CAD build for the part. Positions are in the model's coordinates, mm. A direction names the side the tool comes from. Coordinates: 2 decimals unless noted, no trailing zeros. Order: outer loops, then holes, each group sorted by start corner. A loop starts at its lowest first (then second) coordinate and runs counter-clockwise, first axis right, second up.
from build123d import *

# Parameters (mm, degrees)
SKETCH1_R           = 2.5
BOSS_EXTRUDE1_DEPTH = 3.18
CUT_EXTRUDE1_DEPTH  = 147.499595989
FILLET1_R           = 10


with BuildPart() as part:
    # Sketch1 → Boss-Extrude1 (new body)
    with BuildSketch(Plane(origin=(0, 0, 0), x_dir=(1, 0, 0), z_dir=(0, 1, 0))):
        Polygon((0, 0), (40, 0), (90, 0), (90, 40), (90, 75.550937794), (90, 115.550937794), (-50, 115.550937794), (-50, 0), align=None)
        with Locations(Location((-35, 105.550937794, 0), (0, 0, 90))):
            Circle(SKETCH1_R, mode=Mode.SUBTRACT)
        with Locations(Location((75, 105.550937794, 0), (0, 0, 90))):
            Circle(SKETCH1_R, mode=Mode.SUBTRACT)
        with Locations(Location((20, 85.550937794, 0), (0, 0, 90))):
            Circle(SKETCH1_R, mode=Mode.SUBTRACT)
        with Locations(Location((10, 7.5, 0), (0, 0, 90))):
            Circle(SKETCH1_R, mode=Mode.SUBTRACT)
        with Locations(Location((30, 7.5, 0), (0, 0, 90))):
            Circle(SKETCH1_R, mode=Mode.SUBTRACT)
        with Locations(Location((10, 32, 0), (0, 0, 90))):
            Circle(SKETCH1_R, mode=Mode.SUBTRACT)
        with Locations(Location((30, 32, 0), (0, 0, 90))):
            Circle(SKETCH1_R, mode=Mode.SUBTRACT)
    extrude(amount=BOSS_EXTRUDE1_DEPTH)

    # Sketch3 → Cut-Extrude1 (cut, through all)
    with BuildSketch(Plane.XZ):
        Polygon((90, -75.550937794), (50, -37.231146138), (50, 0), (90, 0), (90, -37.231146138), align=None)
        Polygon((-10, -37.231146138), (-50, -75.550937794), (-50, -37.231146138), (-50, 0), (-10, 0), align=None)
    extrude(amount=-CUT_EXTRUDE1_DEPTH, mode=Mode.SUBTRACT)

    # Fillet1
    fillet1_edges = [part.edges().sort_by_distance(p)[0] for p in [
        (-50, 1.59, -115.550937794),
        (90, 1.59, -115.550937794),
        (90, 1.59, -75.550937794),
        (50, 1.59, -37.231146138),
        (50, 1.59, 0),
        (-10, 1.59, 0),
        (-10, 1.59, -37.231146138),
        (-50, 1.59, -75.550937794),
    ]]
    fillet(fillet1_edges, radius=FILLET1_R)


solid = part.part
1) Two-plate mould, pull along Z, no slides. Class faces 1 (the cylindrical face through (27.52, 1.57, -31.67)), 2 (the flat face through (20, 2, 0)), 3 (the flat face through (-10, 2, -21)): released by +Z, released by -Z, zero draft, split by the parting line, or undercut.
2) Slice it at A-A (x = 30). List the corners of the cut face in (y, z).
3) Which spindle directions (+Z, -Z, +X, -X, +Y, -Y) get a long thin tool onto all of the face, cutting with end or side? Do faces 4 (the flat face through (50, 2, -22)), 5 (the flat face through (-50, 2, -93)). Say none if no direction does.
4) Slice it at C-C (z = -7.5). List the corners of the cut face in (x, y), plus the area to 3 significant figures.
5) Drill centre lines: probe 1 along Z at (x, y) = (30, 2.25); probe 2 along X at (y, z) = (1.7, -32); probe 3 along X at (y, z) = (2.55, -7). Where is each one in solid material? Low to high.
6) Slice it at B-B (y = 2.35). List the corners of the cut face in (x, z).
7) Slice it at D-D (x = -35). List the corners of the cut face in (y, z).
Worked out:
1. face 1: undercut
1. face 2: released by +Z
1. face 3: zero draft
2. outline: (0, -115.55) - (3.18, -115.55) - (3.18, -34.5) - (0, -34.5) - close; (0, -29.5) - (3.18, -29.5) - (3.18, -10) - (0, -10) - close; (0, -5) - (3.18, -5) - (3.18, 0) - (0, 0) - close
3. face 4: +Z, +X, +Y, -Y
3. face 5: +Z, -Z, -X, +Y, -Y
4. outline: (-9.68, 0) - (7.5, 0) - (7.5, 3.18) - (-9.68, 3.18) - close; (12.5, 0) - (27.5, 0) - (27.5, 3.18) - (12.5, 3.18) - close; (32.5, 0) - (49.68, 0) - (49.68, 3.18) - (32.5, 3.18) - close
4. area: 157 mm2
5. probe 1: z = -115.55 to -34.5, -29.5 to -10, -5 to 0
5. probe 2: x = -10 to 7.5, 12.5 to 27.5, 32.5 to 50
5. probe 3: x = -9.54 to 7.55, 12.45 to 27.55, 32.45 to 49.54
6. outline: (-50, -105.55) arc R10 ccw to (-40, -115.55) - (80, -115.55) arc R10 ccw to (90, -105.55) - (90, -79.82) arc R10 ccw to (86.92, -72.6) - (53.08, -40.18) arc R10 cw to (50, -32.96) - (50, -10) arc R10 ccw to (40, 0) - (0, 0) arc R10 ccw to (-10, -10) - (-10, -32.96) arc R10 cw to (-13.08, -40.18) - (-46.92, -72.6) arc R10 ccw to (-50, -79.82) - close; hole circle Ø5 at (-35, -105.55); hole circle Ø5 at (10, -32); hole circle Ø5 at (10, -7.5); hole circle Ø5 at (20, -85.55); hole circle Ø5 at (30, -32); hole circle Ø5 at (30, -7.5); hole circle Ø5 at (75, -105.55)
7. outline: (0, -115.55) - (3.18, -115.55) - (3.18, -108.05) - (0, -108.05) - close; (0, -103.05) - (3.18, -103.05) - (3.18, -61.18) - (0, -61.18) - close
